Source: CAD feature listing. Evaluate the final solid. Frame: model axes, mm. Give positions to 0.01 mm unless a question says otherwise; leave off trailing zeros. Loops run counter-clockwise (first coordinate to the right, second up) from the corner with the lowest first, then second, coordinate; pieces in that order, holes last. Notation, with made-up numbers: M -20,50.5 L 11,50.5 A24 cw 11,85.5 Z; hole C 81.25,65 d6. An arc over 180 degrees is marked long. Write item = value, one per line.
from build123d import *

# Parameters (mm, degrees)
SKETCH_W     = 11.4
SKETCH_H     = 11.4
SKETCH_R     = 1.5
PAD_DEPTH    = 328.85
SKETCH001_R  = 1.5
POCKET_DEPTH = 11.401


with BuildPart() as part:
    # Sketch → Pad (new body)
    with BuildSketch(Plane.XY):
        with Locations((5.7, 5.7)):
            Rectangle(SKETCH_W, SKETCH_H)
        with Locations((5.7, 5.7)):
            Circle(SKETCH_R, mode=Mode.SUBTRACT)
    extrude(amount=PAD_DEPTH)

    # Sketch001 → Pocket (cut, through all)
    with BuildSketch(Plane.YZ.offset(11.4)):
        with Locations((5.7, 39.65)):
            Circle(SKETCH001_R)
        with Locations((5.7, 31.65)):
            Circle(SKETCH001_R)
        with Locations((5.7, 19)):
            Circle(SKETCH001_R)
        with Locations((5.7, 11)):
            Circle(SKETCH001_R)
        with Locations((5.7, 196)):
            Circle(SKETCH001_R)
        with Locations((5.7, 188)):
            Circle(SKETCH001_R)
        with Locations((5.7, 317.85)):
            Circle(SKETCH001_R)
        with Locations((5.7, 309.85)):
            Circle(SKETCH001_R)
    extrude(amount=-POCKET_DEPTH, mode=Mode.SUBTRACT)


solid = part.part
1. Cut plane B-B, the plane z = 155. Return the cut outline in (x, y).
Derived:
outline = M 0,0 L 11.4,0 L 11.4,11.4 L 0,11.4 Z; hole C 5.7,5.7 d3
2. First-contact query: pin 1 Ø3.5 at (x, y) = (5.7, 5.7) entering from -Z; pin 2 Ø2.5 at (y, z) = (5.7, 11) entering from +X. Flat tips, straight axial feed; report the tip coordinate or a pass-through.
Derived:
pin_1 = 0
pin_2 = through
3. Material intervals for probe 1 along Y at (x, z) = (1.5, 196); probe 2 along X at (y, z) = (6, 42.5); probe 3 along X at (y, z) = (5.25, 315), sorted ascending. Write a range as from..to.
Derived:
probe_1 = 0..4.2, 7.2..11.4
probe_2 = 0..4.23, 7.17..11.4
probe_3 = 0..4.27, 7.13..11.4
4. Cut plane A-A, the plane x = 9. Count the separate pieces of the cut face and the enclosed holes in it, then the cut area to 3 significant figures.
Derived:
separate_pieces = 1
enclosed_holes = 8
area = 3,690 mm²
